```python
from build123d import *

# Parameters (mm, degrees)
MAIN_EXTRUSION_DEPTH = 100


with BuildPart() as part:
    # Sk Main Extrusion → Main Extrusion (new body)
    with BuildSketch(Plane.XY):
        with BuildLine():
            Line((-3.83, 2.5328), (-11.31249103, 2.925083334))
            ThreePointArc((-11.31249103, 2.925083334), (-11.819967595, 3.366238681), (-11.514691833, 3.965369062))
            Line((-11.514691833, 3.965369062), (-10.100108722, 4.625))
            Line((-10.100108722, 4.625), (-9.58, 4.3))
            Line((-9.58, 4.3), (-8.08, 4.3))
            Line((-8.08, 4.3), (-5.474147193, 5))
            Line((-5.474147193, 5), (-4.934147193, 5))
            Line((-4.934147193, 5), (-4.23, 4.56))
            Line((-4.23, 4.56), (-4.23, 4.025))
            ThreePointArc((-4.23, 4.025), (-4.112842694, 3.742157269), (-3.829999948, 3.625))
            Line((-3.829999948, 3.625), (1.67, 3.625))
            Line((1.67, 3.625), (1.67, 5.120055168))
            Line((1.67, 5.120055168), (1.19886836, 5.120055168))
            ThreePointArc((1.19886836, 5.120055168), (0.3740485, 5.504367154), (0.038, 6.35))
            Line((0.038, 6.35), (0.038, 6.65))
            ThreePointArc((0.038, 6.65), (0.3740485, 7.495632846), (1.19886836, 7.879944832))
            Line((1.19886836, 7.879944832), (1.67, 7.879944832))
            Line((1.67, 7.879944832), (1.67, 17))
            ThreePointArc((1.67, 17), (1.450330086, 17.530330086), (0.92, 17.75))
            Line((0.92, 17.75), (0.663, 17.75))
            ThreePointArc((0.663, 17.75), (0.038, 18.375), (0.663, 19))
            Line((0.663, 19), (27.295, 19))
            ThreePointArc((27.295, 19), (27.92, 18.375), (27.295, 17.75))
            Line((27.295, 17.75), (25.92, 17.75))
            Line((25.92, 17.75), (25.92, 17.375))
            ThreePointArc((25.92, 17.375), (25.295, 16.75), (24.67, 17.375))
            Line((24.67, 17.375), (24.67, 17.75))
            Line((24.67, 17.75), (3.67, 17.75))
            ThreePointArc((3.67, 17.75), (3.139669914, 17.530330086), (2.92, 17))
            Line((2.92, 17), (2.92, -17))
            ThreePointArc((2.92, -17), (3.139669914, -17.530330086), (3.67, -17.75))
            Line((3.67, -17.75), (24.67, -17.75))
            Line((24.67, -17.75), (24.67, -17.375))
            ThreePointArc((24.67, -17.375), (25.295, -16.75), (25.92, -17.375))
            Line((25.92, -17.375), (25.92, -17.75))
            Line((25.92, -17.75), (27.295, -17.75))
            ThreePointArc((27.295, -17.75), (27.92, -18.375), (27.295, -19))
            Line((27.295, -19), (0.663, -19))
            ThreePointArc((0.663, -19), (0.038, -18.375), (0.663, -17.75))
            Line((0.663, -17.75), (0.92, -17.75))
            ThreePointArc((0.92, -17.75), (1.450330086, -17.530330086), (1.67, -17))
            Line((1.67, -17), (1.67, -7.879944832))
            Line((1.67, -7.879944832), (1.19886836, -7.879944832))
            ThreePointArc((1.19886836, -7.879944832), (0.374048509, -7.495632855), (0.038, -6.650000026))
            Line((0.038, -6.650000026), (0.038, -6.350000026))
            ThreePointArc((0.038, -6.350000026), (0.374048491, -5.504367164), (1.19886836, -5.120055168))
            Line((1.19886836, -5.120055168), (1.67, -5.120055168))
            Line((1.67, -5.120055168), (1.67, -3.625))
            Line((1.67, -3.625), (-3.829999948, -3.625))
            ThreePointArc((-3.829999948, -3.625), (-4.112842694, -3.742157269), (-4.23, -4.025))
            Line((-4.23, -4.025), (-4.23, -4.56))
            Line((-4.23, -4.56), (-4.934147193, -5))
            Line((-4.934147193, -5), (-5.474147193, -5))
            Line((-5.474147193, -5), (-8.08, -4.3))
            Line((-8.08, -4.3), (-9.58, -4.3))
            Line((-9.58, -4.3), (-10.100108722, -4.625))
            Line((-10.100108722, -4.625), (-11.514691833, -3.965369062))
            ThreePointArc((-11.514691833, -3.965369062), (-11.819967595, -3.366238681), (-11.31249103, -2.925083334))
            Line((-11.31249103, -2.925083334), (-3.83, -2.5328))
            Line((-3.83, -2.5328), (1.67, -2.436797143))
            Line((1.67, -2.436797143), (1.67, 2.436797143))
            Line((1.67, 2.436797143), (-3.83, 2.5328))
        make_face()
    extrude(amount=-MAIN_EXTRUSION_DEPTH)


solid = part.part
```
The model under review builds one solid part; all positions refer to its coordinate system, in mm. A direction names the side the tool comes from. Give positions to 0.01 mm unless a question says otherwise; leave off trailing zeros. Order: outer loops, then holes, each group sorted by start corner. A loop starts at its lowest first (then second) coordinate and runs counter-clockwise, first axis right, second up. Notation, with made-up numbers: (71, -27.5) - (103, -27.5) arc R17 ccw to (103, -15.5) - close; hole circle Ø3 at (39.5, 15.25). An arc over 180 degrees is marked (long way). Use CSV: the item, a comma, the result in double quotes. Start each with the question number.
Q1. Tool access review of faces 1 (the flat face through (14, 17.75, -49)), 2 (the flat face through (-7.62, -2.73, -49.3)), 3 (the flat face through (14, 19, -49)), 4 (the flat face through (-6.795, 4.645, -49.3)), 5 (the flat face through (-6.759, -4.655, -49.3)): name each direction out of +Z, -Z, +X, -X, +Y, -Y from which nothing blocks a thin tool from reaching the whole face with its end or side.
Q2. The part is to be moulded in two halves that separate along X. For faces 6 (the flat face through (1.67, 12, -49)), 7 (the flat face through (14, -19, -49)), 8 (the flat face through (-1, -3.625, -49)), say which applies: +X half, -X half, draft (parallel to the pull), parting line (faces both ways), or undercut.
Q3. We need section A-A, the plane x = 17. Write out the cut boundary in (y, z), and give its area (3 significant figures).
Q4. Clearance check with flat-ended pins moving along their axes: pin 1 Ø1 at (y, z) = (-11.5, -28.5) entering from -X; pin 2 Ø5 at (y, z) = (7.5, -58.5) entering from +X; pin 3 Ø8 at (x, y) = (-6.5, -9.5) entering from -Z. State where each tip first meets the part, or that it passes through.
Q5. To check wall thickness, follow line 1 along Y through (x, z) = (21, -48); line 2 along X through (y, z) = (1.5, -49); line 3 along Y through (x, z) = (1.5, -41) (1 decimal). State the ranges of each line that lie inside material, in increasing order. Write a range as [from, to].
Q6. We need section B-B, the plane y = 0. Write out the cut boundary in (x, z), and give its area (3 significant figures).
Outcome:
1,face 1,"+Z, -Z"
1,face 2,"+Z, -Z, -X"
1,face 3,"+Z, -Z, +X, -X, +Y"
1,face 4,"+Z, -Z, +Y"
1,face 5,"+Z, -Z, -Y"
2,face 6,"-X half"
2,face 7,"draft"
2,face 8,"undercut"
3,outline,"(-19, -100) - (-17.75, -100) - (-17.75, 0) - (-19, 0) - close; (17.75, -100) - (19, -100) - (19, 0) - (17.75, 0) - close"
3,area,"250 mm^2"
4,pin 1,"stops at x = 1.67"
4,pin 2,"stops at x = 2.92"
4,pin 3,"passes through"
5,line 1,"y = [-19, -17.75], [17.75, 19]"
5,line 2,"x = [1.67, 2.92]"
5,line 3,"y = [-19, -17.5], [-7.9, -5.1], [-3.6, -2.4], [2.4, 3.6], [5.1, 7.9], [17.5, 19]"
6,outline,"(1.67, -100) - (2.92, -100) - (2.92, 0) - (1.67, 0) - close"
6,area,"125 mm^2"
